Can you work these out from the model? Positions are in its coordinate system, mm. A direction names the side the tool comes from. Give positions to 0.01 mm unless a question says otherwise; leave off trailing zeros. Order: outer loops, then holes, each group sorted by start corner. A loop starts at its lowest first (then second) coordinate and runs counter-clockwise, first axis right, second up. Notation, with made-up numbers: (-6.75, 37.25) - (28.25, 37.25) arc R22 cw to (28.25, 65.25) - close; hole circle Ø1 at (-27, 58.5). An arc over 180 degrees is marked (long way). Answer as a JSON object with one key per item and string values.
```python
from build123d import *

# Parameters (mm, degrees)
CROQUIS1_W              = 88
CROQUIS1_H              = 122.5
SALIENTE_EXTRUIR1_DEPTH = 5
CROQUIS2_W              = 44
CROQUIS2_H              = 74.95
CORTAR_EXTRUIR1_DEPTH   = 5
CROQUIS3_W              = 3
CROQUIS3_H              = 3
SALIENTE_EXTRUIR7_DEPTH = 8
SALIENTE_EXTRUIR8_DEPTH = 38
CROQUIS6_W              = 26
CROQUIS6_H              = 87.95
CORTAR_EXTRUIR3_DEPTH   = 19


with BuildPart() as part:
    # Croquis1 → Saliente-Extruir1 (new body)
    with BuildSketch(Plane(origin=(0, 0, 0), x_dir=(1, 0, 0), z_dir=(0, 1, 0))):
        Rectangle(CROQUIS1_W, CROQUIS1_H)
    extrude(amount=SALIENTE_EXTRUIR1_DEPTH)

    # Croquis2 → Cortar-Extruir1 (cut)
    with BuildSketch(Plane(origin=(0, 5, 0), x_dir=(1, 0, 0), z_dir=(0, 1, 0))):
        Rectangle(CROQUIS2_W, CROQUIS2_H)
    extrude(amount=-CORTAR_EXTRUIR1_DEPTH, mode=Mode.SUBTRACT)

    # Croquis3 → Saliente-Extruir7 (add)
    with BuildSketch(Plane(origin=(0, 5, 0), x_dir=(1, 0, 0), z_dir=(0, 1, 0))):
        with Locations((-14.5, 39.975)):
            Rectangle(CROQUIS3_W, CROQUIS3_H)
        with Locations((-17.5, 39.975)):
            Rectangle(CROQUIS3_W, CROQUIS3_H)
        with Locations((17.5, 39.975)):
            Rectangle(CROQUIS3_W, CROQUIS3_H)
        with Locations((14.5, 39.975)):
            Rectangle(CROQUIS3_W, CROQUIS3_H)
        with Locations((-14.5, -39.975)):
            Rectangle(CROQUIS3_W, CROQUIS3_H)
        with Locations((-17.5, -39.975)):
            Rectangle(CROQUIS3_W, CROQUIS3_H)
        with Locations((17.5, -39.975)):
            Rectangle(CROQUIS3_W, CROQUIS3_H)
        with Locations((14.5, -39.975)):
            Rectangle(CROQUIS3_W, CROQUIS3_H)
    extrude(amount=SALIENTE_EXTRUIR7_DEPTH)

    # Croquis5 → Saliente-Extruir8 (add)
    with BuildSketch(Plane.ZY.offset(19)):
        Polygon((-41.475, 13), (-41.475, 10), (-43.975, 10), align=None)
        Polygon((43.975, 10), (41.475, 13), (41.475, 10), align=None)
    extrude(amount=-SALIENTE_EXTRUIR8_DEPTH)

    # Croquis6 → Cortar-Extruir3 (cut)
    with BuildSketch(Plane(origin=(0, 5, 0), x_dir=(1, 0, 0), z_dir=(0, 1, 0))):
        Rectangle(CROQUIS6_W, CROQUIS6_H)
    extrude(amount=CORTAR_EXTRUIR3_DEPTH, mode=Mode.SUBTRACT)


solid = part.part
```
Q1. If we section it at D-D, the plane x = -16: Please give me the cut outline in (y, z) (3 decimals).
Recorded:
{"outline": "(0, -61.25) - (5, -61.25) - (5, -41.475) - (10, -41.475) - (10, -43.975) - (13, -41.475) - (13, -38.475) - (5, -38.475) - (5, -37.475) - (0, -37.475) - close; (0, 37.475) - (5, 37.475) - (5, 38.475) - (13, 38.475) - (13, 41.475) - (10, 43.975) - (10, 41.475) - (5, 41.475) - (5, 61.25) - (0, 61.25) - close"}
Q2. If we section it at C-C, the plane z = 17: Please give me the cut outline in (x, y), then the cut area to 3 significant figures.
Recorded:
{"outline": "(-44, 0) - (-22, 0) - (-22, 5) - (-44, 5) - close; (22, 0) - (44, 0) - (44, 5) - (22, 5) - close", "area": "220 mm^2"}
Q3. Which directions (+Z, -Z, +X, -X, +Y, -Y) give clear straight access to the entire face, cutting with the end or side of a thin tool? Please do faces 4 (the face through (16, 7, -41.475)), 5 (the face through (-13, 9, -40)), 6 (the face through (16, 9, -38.475)), 7 (the face through (22, 3, 1)), 8 (the face through (-16, 7, 41.475)).
Recorded:
{"face 4": "-Z, +X, -X", "face 5": "+Z, -Z, +Y", "face 6": "+X, -X, +Y", "face 7": "+Y, -Y", "face 8": "+Z, +X, -X"}
Q4. We'd pull the mould along X, two halves only. Please class faces 1 (the face through (-16, 9, 38.475)), 2 (the face through (-13, 9, 40)), 3 (the face through (19, 9, -40)): released by +X, released by -X, zero draft, split by the parting line, or undercut.
Recorded:
{"face 1": "zero draft", "face 2": "undercut", "face 3": "released by +X"}
Q5. I need wall thicknesses on L1, parallel to X at y = 5.5, z = -41; L2, parallel to Z at x = 7, y = 3 (3 decimals); L3, parallel to X at y = 3, z = 30. Which ranges of each line are inside material? Lowest first, please.
Recorded:
{"L1": "x = -19 to -13, 13 to 19", "L2": "z = -61.25 to -37.475, 37.475 to 61.25", "L3": "x = -44 to -22, 22 to 44"}
Q6. I'm going to push flat-ended pins straight in: pin 1 Ø3 at (y, z) = (8, -41.5) entering from +X; pin 2 Ø3 at (x, y) = (-12.5, 7) entering from -Z (3 decimals); pin 3 Ø3 at (x, z) = (-27, -7.5) entering from +Y. Where does each tip first touch, or does it pass through?
Recorded:
{"pin 1": "stops at x = 19", "pin 2": "stops at z = -41.475", "pin 3": "stops at y = 5"}
Q7. If we section it at B-B, the plane y = 3.25: Please give me the cut outline in (x, z) (3 decimals).
Recorded:
{"outline": "(-44, -61.25) - (44, -61.25) - (44, 61.25) - (-44, 61.25) - close; hole (-22, -37.475) - (22, -37.475) - (22, 37.475) - (-22, 37.475) - close"}
Q8. If we section it at A-A, the plane x = 7.5: Please give me the cut outline in (y, z) (3 decimals).
Recorded:
{"outline": "(0, -61.25) - (5, -61.25) - (5, -37.475) - (0, -37.475) - close; (0, 37.475) - (5, 37.475) - (5, 61.25) - (0, 61.25) - close"}
